The model under review builds one solid part; all positions refer to its coordinate system, in mm. A direction names the side the tool comes from. Coordinates: 2 decimals unless noted, no trailing zeros. Loops run counter-clockwise (first coordinate to the right, second up) from the corner with the lowest first, then second, coordinate; pieces in that order, holes last. Notation, with made-up numbers: (44, -28) - (68, -28) arc R12 ccw to (68, -13) - close; hole circle Ø11 at (74, 66). An arc over 180 degrees is marked (long way). Use a Markdown table: item, result. Add a question column.
1) For faces 1 (the flat face through (6, 1, 7)), 2 (the flat face through (27.2, 11.9, 15)), 3 (the flat face through (10, -2, 7)), list the 3-axis set-ups (+Z, -Z, +X, -X, +Y, -Y) from which the entire face can be reached by the end or side of a thin tool; tool diameter is ignored.
2) Add section B-B, the plane y = 23.5. Give the boundary of the cut face in (x, z).
3) Add section C-C, the plane z = 7.5. Give the number of separate pieces and of enclosed holes in the cut face, and give its area (3 significant figures).
4) Add section A-A, the plane y = 34. Give the boundary of the cut face in (x, z) (3 decimals), and give its area (3 significant figures).
5) To check wall thickness, follow L1, parallel to X at y = 53, z = 1.25; L2, parallel to X at y = -1, z = 6.5; L3, parallel to X at y = 70.5, z = 7. State the ranges of each line that lie inside material, in increasing order. Write a range as [from, to].
6) Clearance check with flat-ended pins moving along their axes: pin 1 (1.2 mm diameter, centred on x = 23.5, z = 10, fed in from -Y); pin 2 (5 mm diameter, centred on y = 22, z = 12, fed in from +X); pin 3 (10 mm diameter, centred on x = 18.5, y = 15.5, fed in from -Z); pin 4 (4 mm diameter, centred on y = 17, z = 6, fed in from -X). State where each tip first meets the part, or that it passes through.
7) The part is to be moulded in two halves that separate along X. For faces 4 (the flat face through (22.605, 39.44, 7.395)), 5 (the flat face through (27.2, 11.9, 0)), 6 (the flat face through (7, 28.591, 7)), say which applies: pulls with the +X half, pulls with the -X half, needs draft (parallel to the pull), parting line crosses it, or undercut.
```python
from build123d import *

# Parameters (mm, degrees)
F1_DEPTH = 15


with BuildPart() as f1:
    # F0 (on Top) → F1 (new body)
    with BuildSketch(Plane.XY):
        Polygon((15, 80), (0, 0), (1, 0), (10, 0), (10, 1), (1, 1), (5.234291, 24.591051), (5.593266, 26.591051), (5.95224, 28.591051), (9.9173, 50.682103), (10.186531, 52.182103), (10.455762, 53.682103), (15, 79), (19.544238, 53.682103), (19.813469, 52.182103), (20.0827, 50.682103), (24.04776, 28.591051), (24.406734, 26.591051), (24.765709, 24.591051), (29, 1), (20, 1), (20, 0), (25, 0), (30, 0), align=None)
        with BuildLine():
            Line((1, 0), (0, 0))
            Line((0, 0), (0, -5))
            Line((0, -5), (2.5, -5))
            ThreePointArc((2.5, -5), (5, -2.5), (7.5, -5))
            Line((7.5, -5), (10, -5))
            Line((10, -5), (10, 0))
            Line((10, 0), (1, 0))
        make_face()
        with BuildLine():
            Line((2.5, -5), (0, -5))
            ThreePointArc((0, -5), (1.464466, -8.535534), (5, -10))
            Line((5, -10), (5, -7.5))
            ThreePointArc((5, -7.5), (3.232233, -6.767767), (2.5, -5))
        make_face()
        with BuildLine():
            Line((30, -5), (30, 0))
            Line((30, 0), (25, 0))
            Line((25, 0), (25, -2.5))
            ThreePointArc((25, -2.5), (26.767767, -3.232233), (27.5, -5))
            Line((27.5, -5), (30, -5))
        make_face()
        with BuildLine():
            Line((5, -7.5), (5, -10))
            ThreePointArc((5, -10), (8.535534, -8.535534), (10, -5))
            Line((10, -5), (7.5, -5))
            ThreePointArc((7.5, -5), (6.767767, -6.767767), (5, -7.5))
        make_face()
        with BuildLine():
            Line((25, -2.5), (25, 0))
            Line((25, 0), (20, 0))
            Line((20, 0), (20, -5))
            Line((20, -5), (22.5, -5))
            ThreePointArc((22.5, -5), (23.232233, -3.232233), (25, -2.5))
        make_face()
        with BuildLine():
            ThreePointArc((25, -10), (28.535534, -8.535534), (30, -5))
            Line((30, -5), (27.5, -5))
            ThreePointArc((27.5, -5), (26.767767, -6.767767), (25, -7.5))
            Line((25, -7.5), (25, -10))
        make_face()
        with BuildLine():
            ThreePointArc((20, -5), (21.464466, -8.535534), (25, -10))
            Line((25, -10), (25, -7.5))
            ThreePointArc((25, -7.5), (23.232233, -6.767767), (22.5, -5))
            Line((22.5, -5), (20, -5))
        make_face()
        with BuildLine():
            Line((5.593266, 26.591051), (5.234291, 24.591051))
            Line((5.234291, 24.591051), (7.593266, 24.591051))
            Line((7.593266, 24.591051), (7.593266, 25.591051))
            ThreePointArc((7.593266, 25.591051), (6.886159, 25.883945), (6.593266, 26.591051))
            Line((6.593266, 26.591051), (5.593266, 26.591051))
        make_face()
        with BuildLine():
            Line((5.95224, 28.591051), (5.593266, 26.591051))
            Line((5.593266, 26.591051), (6.593266, 26.591051))
            ThreePointArc((6.593266, 26.591051), (6.886159, 27.298158), (7.593266, 27.591051))
            Line((7.593266, 27.591051), (7.593266, 28.591051))
            Line((7.593266, 28.591051), (5.95224, 28.591051))
        make_face()
        with BuildLine():
            Line((7.593266, 25.591051), (7.593266, 24.591051))
            ThreePointArc((7.593266, 24.591051), (9.007479, 25.176838), (9.593266, 26.591051))
            Line((9.593266, 26.591051), (8.593266, 26.591051))
            ThreePointArc((8.593266, 26.591051), (8.300372, 25.883945), (7.593266, 25.591051))
        make_face()
        with BuildLine():
            Line((8.593266, 26.591051), (9.593266, 26.591051))
            ThreePointArc((9.593266, 26.591051), (9.007479, 28.005265), (7.593266, 28.591051))
            Line((7.593266, 28.591051), (7.593266, 27.591051))
            ThreePointArc((7.593266, 27.591051), (8.300372, 27.298158), (8.593266, 26.591051))
        make_face()
        with BuildLine():
            Line((22.406734, 24.591051), (24.765709, 24.591051))
            Line((24.765709, 24.591051), (24.406734, 26.591051))
            Line((24.406734, 26.591051), (23.406734, 26.591051))
            ThreePointArc((23.406734, 26.591051), (22.406734, 25.591051), (21.406734, 26.591051))
            Line((21.406734, 26.591051), (20.406734, 26.591051))
            ThreePointArc((20.406734, 26.591051), (20.992521, 25.176838), (22.406734, 24.591051))
        make_face()
        with BuildLine():
            Line((10.186531, 52.182103), (9.9173, 50.682103))
            Line((9.9173, 50.682103), (11.686531, 50.682103))
            Line((11.686531, 50.682103), (11.686531, 51.182103))
            ThreePointArc((11.686531, 51.182103), (10.979424, 51.474996), (10.686531, 52.182103))
            Line((10.686531, 52.182103), (10.186531, 52.182103))
        make_face()
        with BuildLine():
            Line((23.406734, 26.591051), (24.406734, 26.591051))
            Line((24.406734, 26.591051), (24.04776, 28.591051))
            Line((24.04776, 28.591051), (22.406734, 28.591051))
            ThreePointArc((22.406734, 28.591051), (20.992521, 28.005265), (20.406734, 26.591051))
            Line((20.406734, 26.591051), (21.406734, 26.591051))
            ThreePointArc((21.406734, 26.591051), (22.406734, 27.591051), (23.406734, 26.591051))
        make_face()
        with BuildLine():
            Line((10.455762, 53.682103), (10.186531, 52.182103))
            Line((10.186531, 52.182103), (10.686531, 52.182103))
            ThreePointArc((10.686531, 52.182103), (10.979424, 52.88921), (11.686531, 53.182103))
            Line((11.686531, 53.182103), (11.686531, 53.682103))
            Line((11.686531, 53.682103), (10.455762, 53.682103))
        make_face()
        with BuildLine():
            Line((11.686531, 51.182103), (11.686531, 50.682103))
            ThreePointArc((11.686531, 50.682103), (12.747191, 51.121443), (13.186531, 52.182103))
            Line((13.186531, 52.182103), (12.686531, 52.182103))
            ThreePointArc((12.686531, 52.182103), (12.393638, 51.474996), (11.686531, 51.182103))
        make_face()
        with BuildLine():
            Line((12.686531, 52.182103), (13.186531, 52.182103))
            ThreePointArc((13.186531, 52.182103), (12.747191, 53.242763), (11.686531, 53.682103))
            Line((11.686531, 53.682103), (11.686531, 53.182103))
            ThreePointArc((11.686531, 53.182103), (12.393638, 52.88921), (12.686531, 52.182103))
        make_face()
        with BuildLine():
            Line((18.313469, 50.682103), (20.0827, 50.682103))
            Line((20.0827, 50.682103), (19.813469, 52.182103))
            Line((19.813469, 52.182103), (19.313469, 52.182103))
            ThreePointArc((19.313469, 52.182103), (18.313469, 51.182103), (17.313469, 52.182103))
            Line((17.313469, 52.182103), (16.813469, 52.182103))
            ThreePointArc((16.813469, 52.182103), (17.252809, 51.121443), (18.313469, 50.682103))
        make_face()
        with BuildLine():
            Line((19.313469, 52.182103), (19.813469, 52.182103))
            Line((19.813469, 52.182103), (19.544238, 53.682103))
            Line((19.544238, 53.682103), (18.313469, 53.682103))
            ThreePointArc((18.313469, 53.682103), (17.252809, 53.242763), (16.813469, 52.182103))
            Line((16.813469, 52.182103), (17.313469, 52.182103))
            ThreePointArc((17.313469, 52.182103), (18.313469, 53.182103), (19.313469, 52.182103))
        make_face()
    extrude(amount=F1_DEPTH)


solid = f1.part
```
From the geometry:
| question | item | result |
|---|---|---|
| 1 | face 1 | +Z, -Z |
| 1 | face 2 | +Z, +X, -X, +Y, -Y |
| 1 | face 3 | +Z, -Z, -Y |
| 2 | outline | (4.41, 0) - (5.04, 0) - (5.04, 15) - (4.41, 15) - close; (24.96, 0) - (25.59, 0) - (25.59, 15) - (24.96, 15) - close |
| 3 | separate pieces | 1 |
| 3 | enclosed holes | 6 |
| 3 | area | 269 mm^2 |
| 4 | outline | (6.375, 0) - (6.923, 0) - (6.923, 15) - (6.375, 15) - close; (23.077, 0) - (23.625, 0) - (23.625, 15) - (23.077, 15) - close |
| 4 | area | 16.4 mm^2 |
| 5 | L1 | x = [9.94, 11.11], [12.26, 12.94], [17.06, 17.74], [18.89, 20.06] |
| 5 | L2 | x = [0, 10], [20, 30] |
| 5 | L3 | x = [13.22, 13.47], [16.53, 16.78] |
| 6 | pin 1 | stops at y = -9.92 |
| 6 | pin 2 | stops at x = 26.34 |
| 6 | pin 3 | passes through |
| 6 | pin 4 | stops at x = 2.81 |
| 7 | face 4 | pulls with the +X half |
| 7 | face 5 | needs draft |
| 7 | face 6 | undercut |
